Here's how the part is built. I have some questions about the finished solid (model axes, mm). A direction names the side the tool comes from. Coordinates: 2 decimals unless noted, no trailing zeros. Write each loop counter-clockwise with the first axis right and the second up, starting at its lowest first coordinate (ties: lowest second). Pieces come first, ordered by that corner, then holes. Notation, with made-up numbers: M 35,-24.75 L 67,-24.75 A22 cw 67,-14.75 Z; hole C 31.25,18.25 d3. An arc over 180 degrees is marked long. Use one line per item in the form item = value. Start each with the question number.
1. Thinking about a two-plate mould opening in X: for faces 1 (the face through (-3, 13.899, 9)), 2 (the face through (-9.163, 3, 37)), 3 (the face through (-14.81, 2.02, 38.44)), which applies, released by +X, released by -X, zero draft, split by the parting line, or undercut?
2. On a 3-axis mill with a long thin cutter (end or side, diameter ignored), from which of +Z, -Z, +X, -X, +Y, -Y can I reach the whole of each face in a straight line? I mean faces 4 (the face through (-7.9, 18.5, 71.6)), 5 (the face through (-27.334, 43.307, 66.542)), 6 (the face through (-3, 13.899, 66)). Say none if no direction works.
3. I want a section at D-D, the plane y = 27. List the corners of the cut face in (x, z) for me, plus the area to 3 significant figures.
4. I want a section at A-A, the plane y = 36. List the corners of the cut face in (x, z) for me.
5. Please list where these lines run through material, in increasing order: line 1 along X through (y, z) = (1.4, 37.5); line 2 along X through (y, z) = (5.95, 37.5); line 3 along Z through (x, y) = (-47.5, 30.5). Write a range as [from, to].
6. I'm going to push flat-ended pins straight in: pin 1 Ø12.5 at (x, y) = (-8.5, 21.5) entering from -Z; pin 2 Ø1.5 at (x, z) = (-3, 8.5) entering from +Y; pin 3 Ø3 at (x, z) = (-45.5, 37.5) entering from +Y; pin 4 Ø7.5 at (y, z) = (2.5, 44.5) entering from +X. Where does each tip first touch, or does it pass through?
7. I want a section at C-C, the plane x = -29. List the corners of the cut face in (y, z) for me, plus the area to 3 significant figures.
8. I want a section at B-B, the plane z = 37.5. List the corners of the cut face in (x, y) for me, plus the area to 3 significant figures.
from build123d import *

# Parameters (mm, degrees)
BOSS_EXTRU_1_DEPTH                                 = 5.5
ESQUISSE1_3_R                                      = 1.8
BOSS_EXTRU_2_DEPTH                                 = 6.5
BOSS_EXTRU_3_DEPTH                                 = 11.5
ESQUISSE1_6_W                                      = 41.878391759
ESQUISSE1_6_H                                      = 7.003105655
BOSS_EXTRU_4_DEPTH                                 = 63.5
CHAMBRAGE_POUR_VIS_SIX_PANS_CREUX_M2_5_D           = 3.1
CHAMBRAGE_POUR_VIS_SIX_PANS_CREUX_M2_5_CBORE_D     = 5.5
CHAMBRAGE_POUR_VIS_SIX_PANS_CREUX_M2_5_CBORE_DEPTH = 2.9
CHAMBRAGE_POUR_VIS_SIX_PANS_CREUX_M31_D            = 3.6
CHAMBRAGE_POUR_VIS_SIX_PANS_CREUX_M31_CBORE_D      = 6.5
CHAMBRAGE_POUR_VIS_SIX_PANS_CREUX_M31_CBORE_DEPTH  = 3.4


with BuildPart() as part:
    # Esquisse1 → Boss.-Extru.1 (new body)
    with BuildSketch(Plane.XY):
        Polygon((-51.041668631, 61.918561392), (-51.041668631, 57.051835463), (-12.364240457, 19.369216184), (-7.689286801, 24.167587096), (-46.436874542, 61.918561392), align=None)
    extrude(amount=BOSS_EXTRU_1_DEPTH)



with BuildPart() as body_2:
    # Esquisse1_3 → Boss.-Extru.2 (new body)
    with BuildSketch(Plane.XY):
        Polygon((-6.8709698, 13.899199983), (0, 13.899199983), (0, 20.573191179), (-4.963123823, 25.408660192), (-5.800119712, 24.549567884), (-5.832093395, 24.580719183), (-11.676946527, 18.581563828), align=None)
        with Locations(Location((-6.5, 19.899199983, 0), (0, 0, 180))):
            Circle(ESQUISSE1_3_R, mode=Mode.SUBTRACT)
    extrude(amount=BOSS_EXTRU_2_DEPTH)


with BuildPart() as part_1:
    add(part.part)

    add(body_2.part)  # Boss.-Extru.3 merges body 2
    # Esquisse1_5 → Boss.-Extru.3 (add)
    with BuildSketch(Plane.XY):
        Polygon((-9.163276872, 0), (0, 0), (0, 13.899199983), (-6.8709698, 13.899199983), (-11.676946527, 18.581563828), (-5.832093395, 24.580719183), (-5.800119712, 24.549567884), (-4.963123823, 25.408660192), (-42.436874542, 61.918561392), (-46.436874542, 61.918561392), (-7.689286801, 24.167587096), (-12.364240457, 19.369216184), (-51.041668631, 57.051835463), (-51.041668631, 7.003105655), (-9.163276872, 7.003105655), align=None)
    extrude(amount=BOSS_EXTRU_3_DEPTH)

    # Esquisse1_6 → Boss.-Extru.4 (add)
    with BuildSketch(Plane.XY):
        with Locations((-30.102472752, 3.501552828)):
            Rectangle(ESQUISSE1_6_W, ESQUISSE1_6_H)
    extrude(amount=BOSS_EXTRU_4_DEPTH)

    # Sym_trie2: part across plane


with BuildPart() as part_2:
    add(part_1.part)
    add(part_1.part.mirror(Plane.XY.offset(37.5)))

    # Chambrage pour vis _ six pans creux M2.5 (through all)
    with Locations(Plane(origin=(0, 7.003105655, 0), x_dir=(1, 0, 0), z_dir=(0, 1, 0))):
        with Locations((-45.041668631, -37.5), (-16.041668631, -37.5)):
            CounterBoreHole(CHAMBRAGE_POUR_VIS_SIX_PANS_CREUX_M2_5_D / 2, CHAMBRAGE_POUR_VIS_SIX_PANS_CREUX_M2_5_CBORE_D / 2, CHAMBRAGE_POUR_VIS_SIX_PANS_CREUX_M2_5_CBORE_DEPTH)

    # Chambrage pour vis _ six pans creux M31 (through all)
    with Locations(Plane(origin=(0, 0, 0), x_dir=(-1, 0, 0), z_dir=(0, 0, -1))):
        with Locations((6.5, 19.899199983)):
            chambrage_pour_vis_six_pans_creux_m31 = CounterBoreHole(CHAMBRAGE_POUR_VIS_SIX_PANS_CREUX_M31_D / 2, CHAMBRAGE_POUR_VIS_SIX_PANS_CREUX_M31_CBORE_D / 2, CHAMBRAGE_POUR_VIS_SIX_PANS_CREUX_M31_CBORE_DEPTH)

    # Sym_trie3: Chambrage pour vis _ six pans creux M31 across plane
    add(chambrage_pour_vis_six_pans_creux_m31.mirror(Plane.XY.offset(37.5)), mode=Mode.SUBTRACT)


solid = part_2.part
Answer list:
q1.face_1 = zero draft
q1.face_2 = released by +X
q1.face_3 = undercut
q2.face_4 = +Z
q2.face_5 = none
q2.face_6 = +X
q3.outline = M -51.04,0 L -6.6,0 L -6.6,11.5 L -10.6,11.5 L -10.6,5.5 L -20.2,5.5 L -20.2,11.5 L -51.04,11.5 Z; M -51.04,63.5 L -20.2,63.5 L -20.2,69.5 L -10.6,69.5 L -10.6,63.5 L -6.6,63.5 L -6.6,75 L -51.04,75 Z
q3.area = 907 mm²
q4.outline = M -51.04,0 L -15.83,0 L -15.83,11.5 L -19.83,11.5 L -19.83,5.5 L -29.43,5.5 L -29.43,11.5 L -51.04,11.5 Z; M -51.04,63.5 L -29.43,63.5 L -29.43,69.5 L -19.83,69.5 L -19.83,63.5 L -15.83,63.5 L -15.83,75 L -51.04,75 Z
q5.line_1 = [-51.04, -46.59], [-43.49, -17.59], [-14.49, -9.16]
q5.line_2 = [-51.04, -47.79], [-42.29, -18.79], [-13.29, -9.16]
q5.line_3 = [0, 11.5], [63.5, 75]
q6.pin_1 = 0
q6.pin_2 = 13.9
q6.pin_3 = 4.1
q6.pin_4 = -9.16
q7.outline = M 0,0 L 48.83,0 L 48.83,11.5 L 44.93,11.5 L 44.93,5.5 L 35.58,5.5 L 35.58,11.5 L 7,11.5 L 7,63.5 L 35.58,63.5 L 35.58,69.5 L 44.93,69.5 L 44.93,63.5 L 48.83,63.5 L 48.83,75 L 0,75 Z
q7.area = 1,370 mm²
q8.outline = M -51.04,0 L -46.59,0 L -46.59,4.1 L -47.79,4.1 L -47.79,7 L -51.04,7 Z; M -43.49,0 L -17.59,0 L -17.59,4.1 L -18.79,4.1 L -18.79,7 L -42.29,7 L -42.29,4.1 L -43.49,4.1 Z; M -14.49,0 L -9.16,0 L -9.16,7 L -13.29,7 L -13.29,4.1 L -14.49,4.1 Z
q8.area = 236 mm²
